Could you check a few things on this model? Use its own coordinates, in mm. A direction names the side the tool comes from. Give positions to 0.01 mm unless a question says otherwise; leave off trailing zeros. Order: outer loops, then holes, each group sorted by start corner. A loop starts at its lowest first (then second) coordinate and runs counter-clockwise, first axis right, second up.
from build123d import *

# Parameters (mm, degrees)
BOSS_EXTRUDE1_DEPTH = 90
WRAP1_START         = -6.633249581
WRAP1_OUTLINE_W     = 6
WRAP1_OUTLINE_H     = 6
WRAP1_DEPTH         = 6.633249581
SKETCH4_W           = 3.6
SKETCH4_H           = 8
CUT_EXTRUDE1_DEPTH  = 5
CIRPATTERN3_COUNT   = 2
BOSS_EXTRUDE2_DEPTH = 2
LPATTERN1_COUNT     = 6
LPATTERN1_PITCH     = 14
BOSS_EXTRUDE3_DEPTH = 6
FILLET4_R           = 3.2


# Read off the part's stored shape, not the designer's step: Wrap1
with BuildPart() as part:
    # Sketch1 → Boss-Extrude1 (new body)
    with BuildSketch(Plane(origin=(0, 0, 0), x_dir=(1, 0, 0), z_dir=(0, 1, 0))):
        with BuildLine():
            Line((-3.31662479, 5), (-3.31662479, -5))
            ThreePointArc((-3.31662479, -5), (0, -6), (3.31662479, -5))
            Line((3.31662479, -5), (3.31662479, 5))
            ThreePointArc((3.31662479, 5), (0, 6), (-3.31662479, 5))
        make_face()
        with BuildLine():
            Line((-1.81662479, -4.658312395), (-1.81662479, 4.658312395))
            ThreePointArc((-1.81662479, 4.658312395), (0, 5), (1.81662479, 4.658312395))
            Line((1.81662479, 4.658312395), (1.81662479, -4.658312395))
            ThreePointArc((1.81662479, -4.658312395), (0, -5), (-1.81662479, -4.658312395))
        make_face(mode=Mode.SUBTRACT)
    extrude(amount=BOSS_EXTRUDE1_DEPTH)

    # Wrap1 outline → Wrap1 (cut)
    with BuildSketch(Plane(origin=(3.31662479, 0, 0), x_dir=(0, 0, -1), z_dir=(1, 0, 0)).offset(WRAP1_START)):
        with Locations((0, 79)):
            Rectangle(WRAP1_OUTLINE_W, WRAP1_OUTLINE_H)
        with Locations((0, 65)):
            Rectangle(WRAP1_OUTLINE_W, WRAP1_OUTLINE_H)
        with Locations((0, 51)):
            Rectangle(WRAP1_OUTLINE_W, WRAP1_OUTLINE_H)
        with Locations((0, 37)):
            Rectangle(WRAP1_OUTLINE_W, WRAP1_OUTLINE_H)
        with Locations((0, 23)):
            Rectangle(WRAP1_OUTLINE_W, WRAP1_OUTLINE_H)
        with Locations((0, 9)):
            Rectangle(WRAP1_OUTLINE_W, WRAP1_OUTLINE_H)
    extrude(amount=WRAP1_DEPTH, mode=Mode.SUBTRACT)

    # Sketch4 → Cut-Extrude1 (cut)
    with BuildSketch(Plane.XY.offset(6)):
        with Locations((0, 10)):
            Rectangle(SKETCH4_W, SKETCH4_H)
        with Locations((0, 24)):
            Rectangle(SKETCH4_W, SKETCH4_H)
        with Locations((0, 38)):
            Rectangle(SKETCH4_W, SKETCH4_H)
        with Locations((0, 52)):
            Rectangle(SKETCH4_W, SKETCH4_H)
        with Locations((0, 66)):
            Rectangle(SKETCH4_W, SKETCH4_H)
        with Locations((0, 80)):
            Rectangle(SKETCH4_W, SKETCH4_H)
    cut_extrude1 = extrude(amount=-CUT_EXTRUDE1_DEPTH, mode=Mode.SUBTRACT)

    # CirPattern3: Cut-Extrude1 ×2 about axis
    cirpattern3_axis = Axis((0, 90, 0), (0, -1, 0))
    for i in range(1, CIRPATTERN3_COUNT):
        add(cut_extrude1.rotate(cirpattern3_axis, i * 360 / CIRPATTERN3_COUNT), mode=Mode.SUBTRACT)

    # Sketch5 → Boss-Extrude2 (add)
    with BuildSketch(Plane.XZ):
        with BuildLine():
            Line((1.81662479, 4.658312395), (1.81662479, -4.658312395))
            ThreePointArc((1.81662479, -4.658312395), (0, -5), (-1.81662479, -4.658312395))
            Line((-1.81662479, -4.658312395), (-1.81662479, 4.658312395))
            ThreePointArc((-1.81662479, 4.658312395), (0, 5), (1.81662479, 4.658312395))
        make_face()
    extrude(amount=-BOSS_EXTRUDE2_DEPTH)

    # Sketch8 → Loft1 section 0
    with BuildSketch(Plane.ZY.offset(-1.81662479)):
        with BuildLine():
            Line((-2, 75), (2, 75))
            Line((2, 75), (2, 73.5))
            Line((2, 73.5), (-2, 73.5))
            Line((-2, 73.5), (-2, 75))
        make_face()
    # Sketch6 → Loft1 section 1
    with BuildSketch(Plane(origin=(-1.81662479, 0, 0), x_dir=(0, 0, -1), z_dir=(1, 0, 0))):
        with BuildLine():
            Line((-2, 84.5), (2, 84.5))
            Line((2, 84.5), (2, 83))
            Line((2, 83), (-2, 83))
            Line((-2, 83), (-2, 84.5))
        make_face()
    loft1 = loft()

    # LPattern1: Loft1 ×6
    with Locations(*[(0, -i * LPATTERN1_PITCH, 0) for i in range(1, LPATTERN1_COUNT)]):
        add(loft1)

    # Sketch10 → Boss-Extrude3 (add)
    with BuildSketch(Plane(origin=(0, 90, 0), x_dir=(1, 0, 0), z_dir=(0, 1, 0))):
        with BuildLine():
            Line((-3.31662479, 5), (-3.31662479, -5))
            ThreePointArc((-3.31662479, -5), (0, -6), (3.31662479, -5))
            Line((3.31662479, -5), (3.31662479, 5))
            ThreePointArc((3.31662479, 5), (0, 6), (-3.31662479, 5))
        make_face()
    extrude(amount=BOSS_EXTRUDE3_DEPTH)

    # Fillet4
    # the kernel refuses this fillet: 3.2 mm, written as the material it takes off along each edge
    with BuildSketch(Plane(origin=(0, 96, 0), x_dir=(0.9398790484692316, 0, 0.34150750247772244), z_dir=(-0.34150750247772244, 0, 0.9398790484692316))) as fillet4_piece_1:
        with BuildLine():
            CenterArc((6 - FILLET4_R, -FILLET4_R), FILLET4_R, 0, 90)
            Line((6, -FILLET4_R), (6, 0))
            Line((6, 0), (6 - FILLET4_R, 0))
        make_face()
    revolve(axis=Axis((0, 96, 0), (0, 1, 0)), revolution_arc=219.937491809, mode=Mode.SUBTRACT)
    with BuildSketch(Plane(origin=(-3.31662479, 96, -13), x_dir=(0, -1, 0), z_dir=(0, 0, 1)), Plane(origin=(3.31662479, 96, 13), x_dir=(0, -1, 0), z_dir=(0, 0, -1))) as fillet4_piece_2:
        with BuildLine():
            CenterArc((FILLET4_R, FILLET4_R), FILLET4_R, 180, 90)
            Line((0, FILLET4_R), (0, 0))
            Line((0, 0), (FILLET4_R, 0))
        make_face()
    extrude(amount=26, mode=Mode.SUBTRACT)
    with BuildSketch(Plane(origin=(0, 96, 0), x_dir=(-0.9398790484692316, 0, -0.34150750247772244), z_dir=(0.34150750247772244, 0, -0.9398790484692316))) as fillet4_piece_3:
        with BuildLine():
            CenterArc((6 - FILLET4_R, -FILLET4_R), FILLET4_R, 0, 90)
            Line((6 - FILLET4_R, 0), (6, 0))
            Line((6, 0), (6, -FILLET4_R))
        make_face()
    revolve(axis=Axis((0, 96, 0), (0, 1, 0)), revolution_arc=219.937491809, mode=Mode.SUBTRACT)


solid = part.part
Item 1: For faces 1 (the flat face through (3, 40, 0)), 2 (the flat face through (-3, 12, 0)), 3 (the flat face through (-3, 65, 3)), 4 (the flat face through (-0.025, 50.317, 0.028)), which set-ups out of +Z, -Z, +X, -X, +Y, -Y let a thin tool reach every point of the face, with its end or its side?
Findings:
face 1: +X
face 2: -X
face 3: +X, -X
face 4: none
Item 2: For pin 1 (1.2 mm diameter, centred on x = 2.5, y = 50, fed in from -Z); pin 2 (1.6 mm diameter, centred on x = 3, y = 66.5, fed in from +Z); pin 3 (1.5 mm diameter, centred on y = 65.5, z = 2.5, fed in from -X); pin 4 (0.7 mm diameter, centred on x = -0.5, z = 5.5, fed in from +Y), each with a flat end and sliding along its axis, tell me the tip position at first contact or that it passes through.
Findings:
pin 1: stops at z = -5.69
pin 2: stops at z = 5.58
pin 3: stops at x = -3.32
pin 4: stops at y = 94.95
Item 3: We'd pull the mould along Z, two halves only. Please class faces 5 (the cylindrical face through (0, 46, 6)), 6 (the flat face through (-3, 68, 0)), 7 (the cylindrical face through (2.35, 95.09, 0.07)): +Z half, -Z half, draft (parallel to the pull), parting line (faces both ways), or undercut.
Findings:
face 5: +Z half
face 6: undercut
face 7: draft
Item 4: Please list where these lines run through material, in increasing order: line 1 along X through (y, z) = (74.5, 3.25); line 2 along Z through (x, y) = (3.25, 39); line 3 along Z through (x, y) = (0.5, 31.5).
Findings:
line 1: x = -3.32 to -1.82, 1.82 to 3.32
line 2: z = -5.04 to -3, 3 to 5.04
line 3: z = -5.98 to -4.97, 4.97 to 5.98
Item 5: Imagine slicing it at B-B on x = 1. Give the number of separate pieces and of enclosed holes in the cut face, then the cut area to 3 significant figures.
Findings:
separate pieces: 18
enclosed holes: 0
area: 207 mm2
Item 6: Imagine slicing it at A-A on y = 44. List the corners of the cut face in (x, z) for me, then the cut area to 3 significant figures.
Findings:
outline: (-3.32, -5) arc R6 ccw to (3.32, -5) - (3.32, 5) arc R6 ccw to (-3.32, 5) - close; hole (-1.82, -4.66) arc R5 ccw to (1.82, -4.66) - (1.82, 4.66) arc R5 ccw to (-1.82, 4.66) - close
area: 39.8 mm2
